The listing builds one solid part. Answer for the finished solid, in the listing's coordinates (mm). A direction names the side the tool comes from. Round coordinates to 2 decimals unless told otherwise and drop trailing zeros. Write each loop counter-clockwise with the first axis right and the second up, starting at its lowest first coordinate (ties: lowest second). Pieces come first, ordered by that corner, then holes. Notation, with made-up numbers: (41, 59) - (56, 59) arc R26 ccw to (56, 93) - close; hole circle Ø4 at (-15.75, 4.5). An arc over 180 degrees is marked (long way). Answer as CSV lines item,"result". Start each with the question number.
Item 1: A cutting plane is placed at B-B on x = -40.5. Determine the outline of the cut face in (y, z), and give its area (3 significant figures).
Item 2: Which of the six approach directions +Z, -Z, +X, -X, +Y, -Y give full straight-line access (tool end or side, diameter ignored) to faces 5 (the flat face through (-63.759, -13, 8)), 6 (the flat face through (-12.57, -38, 13)), 7 (the cylindrical face through (-37.41, -36.33, 58.15))?
Item 3: Flat-ended cylindrical pins translate along their axes: pin 1 (4 mm diameter, centred on y = -35, z = 29, fed in from -X); pin 2 (2 mm diameter, centred on y = -24, z = 33, fed in from +X); pin 3 (5.5 mm diameter, centred on y = -40.5, z = -11.5, fed in from -X). Find the tip coordinate at first contact, or state that the pin passes through.
Item 4: A cutting plane is placed at D-D on x = 11. Determine the outline of the cut face in (y, z), and give its area (3 significant figures).
Item 5: Straight lines are drawn through the part: line 1 along X through (y, z) = (-48, -4); line 2 along Z through (x, y) = (-36, -39); line 3 along Z through (x, y) = (-33.5, -28). For each, find the intervals that lie inside material, in ascending order. Write a range as [from, to].
Item 6: For a pull along Z with two mould halves and no side action, classify faces 1 (the flat face through (63.299, -19, -12)), 2 (the flat face through (-1, -13, -17.831)), 3 (the flat face through (20.952, -12.522, 23.494)), 4 (the flat face through (-26, -25.4, 29)) as pulls with the +Z half, pulls with the -Z half, needs draft (parallel to the pull), parting line crosses it, or undercut.
Item 7: A cutting plane is placed at C-C on z = 36. Determine the outline of the cut face in (x, y), and give its area (3 significant figures).
Item 8: A cutting plane is placed at A-A on y = -35. Determine the outline of the cut face in (x, z), and give its area (3 significant figures).
```python
from build123d import *

# Parameters (mm, degrees)
F0_R     = 12.7
F1_DEPTH = 25.4
F2_R     = 12.7
F3_DEPTH = 50.8
F4_R     = 12.7


with BuildPart() as f1:
    # F0 (on Front) → F1 (new body)
    with BuildSketch(Plane.XZ):
        with BuildLine():
            Line((63.240985, -5.1308), (-24.121142, 54.003528))
            ThreePointArc((-24.121142, 54.003528), (-50.265274, 55.405799), (-63.759015, 32.9692))
            Line((-63.759015, 32.9692), (-63.759015, -17.8308))
            Line((-63.759015, -17.8308), (63.240985, -17.8308))
            Line((63.240985, -17.8308), (63.240985, -5.1308))
        make_face()
        with Locations((-38.359015, 32.9692)):
            Circle(F0_R, mode=Mode.SUBTRACT)
    extrude(amount=F1_DEPTH)

    # F2 (on Front) → F3 (join)
    with BuildSketch(Plane.XZ):
        with BuildLine():
            Line((-12.569834, -5.744165), (-12.569834, 32.757161))
            ThreePointArc((-12.569834, 32.757161), (-37.969834, 58.157161), (-63.369834, 32.757161))
            Line((-63.369834, 32.757161), (-63.700385, -5.744165))
            Line((-63.700385, -5.744165), (-63.700385, -17.234586))
            Line((-63.700385, -17.234586), (63.299008, -17.234586))
            Line((63.299008, -17.234586), (63.299008, -5.744165))
            Line((63.299008, -5.744165), (-12.569834, -5.744165))
        make_face()
        with Locations((-37.969834, 32.757161)):
            Circle(F2_R, mode=Mode.SUBTRACT)
    extrude(amount=F3_DEPTH)

    # F4
    f4_edges = [f1.edges().sort_by_distance(p)[0] for p in [
        (63.299008, -50.8, -11.489375),
    ]]
    fillet(f4_edges, radius=F4_R)


solid = f1.part
```
Geometry says:
1,outline,"(-50.8, -17.23) - (-25.4, -17.23) - (-25.4, -17.83) - (0, -17.83) - (0, 20.45) - (-25.4, 20.45) - (-25.4, 20.31) - (-50.8, 20.31) - close; (-50.8, 45.2) - (0, 45.2) - (0, 58.28) - (-25.4, 58.28) - (-25.4, 58.03) - (-50.8, 58.03) - close"
1,area,"2,580 mm^2"
2,face 5,"+Z, -Z, -X, +Y, -Y"
2,face 6,"+Z, +X, -Y"
2,face 7,"+Z, -Y"
3,pin 1,"stops at x = -63.42"
3,pin 2,"stops at x = 8.39"
3,pin 3,"stops at x = -63.7"
4,outline,"(-50.8, -17.23) - (-25.4, -17.23) - (-25.4, -17.83) - (0, -17.83) - (0, 30.23) - (-25.4, 30.23) - (-25.4, -5.74) - (-50.8, -5.74) - close"
4,area,"1,510 mm^2"
5,line 1,"x = [-63.69, -12.57]"
5,line 2,"z = [-17.23, 20.21], [45.3, 58.08]"
5,line 3,"z = [-17.23, 20.87], [44.64, 57.76]"
6,face 1,"needs draft"
6,face 2,"pulls with the -Z half"
6,face 3,"pulls with the +Z half"
6,face 4,"undercut"
7,outline,"(-63.58, -25.4) - (-63.16, -25.4) - (-63.16, -50.8) - (-50.25, -50.8) - (-50.25, 0) - (-63.58, 0) - close; (-26.03, -25.4) - (-25.69, -25.4) - (-25.69, -50.8) - (-12.78, -50.8) - (-12.78, -25.4) - (2.48, -25.4) - (2.48, 0) - (-26.03, 0) - close"
7,area,"1,720 mm^2"
8,outline,"(-63.7, -17.23) - (63.3, -17.23) - (63.3, -5.74) - (-12.57, -5.74) - (-12.57, 32.76) arc R25.4 ccw to (-63.37, 32.76) - (-63.7, -5.74) - close; hole circle Ø25.4 at (-37.97, 32.76)"
8,area,"3,930 mm^2"
